Autodesk Inventor part; units mm, degrees
ref_plane "YZ Plane" through (0, 0, 0) normal (1, 0, 0) x (0, 1, 0)
ref_plane "XZ Plane" through (0, 0, 0) normal (0, 1, 0) x (-1, 0, 0)
ref_plane "XY Plane" through (0, 0, 0) normal (0, 0, 1) x (1, 0, 0)
sketch "Sketch1" plane through (0, 0, 0) normal (0, 1, 0) x (-1, 0, 0)
  line L0 (32.65, 55) -> (-32.65, 55)
  line L1 (-32.65, 55) -> (-32.65, -55)
  line L2 (-32.65, -55) -> (32.65, -55)
  line L3 (32.65, -55) -> (32.65, 55)
  line L4 (32.65, 55) -> (-32.65, -55) construction
  line L5 (-32.65, 55) -> (32.65, -55) construction
  circle A0 centre (-24.15, 38) radius 1.75
  circle A1 centre (-24.15, -45) radius 1.75
  circle A2 centre (24.15, 37) radius 1.75
  circle A3 centre (24.15, -38) radius 1.75
  point P0 (0, 0)
  dimension "d0" = 110
  dimension "d1" = 65.3
  dimension "d2" = 83
  dimension "d3" = 8.5
  dimension "d4" = 17
  dimension "d5" = 3.5
  dimension "d6" = 3.5
  dimension "d7" = 3.5
  dimension "d8" = 1
  dimension "d9" = 48.3
  dimension "d10" = 3.5
  dimension "d11" = 75
extrude "Extrusion1" add sketch "Sketch1" along normal blind 2
sketch "Sketch2" plane through (-32.65, 0, 55) normal (0, 0, 1) x (1, 0, 0)
  line L0 (0, 70) -> (65.3, 70)
  line L1 (65.3, 70) -> (65.3, 0)
  line L2 (65.3, 0) -> (0, 0)
  line L3 (0, 0) -> (0, 70)
  line L4 (0, 70) -> (65.3, 0) construction
  line L5 (65.3, 70) -> (0, 0) construction
  line L6 (65.3, 0) -> (65.3, 2)
  line L7 (16, 7.5) -> (24.5, 7.5)
  line L8 (24.5, 7.5) -> (24.5, 4)
  line L9 (24.5, 4) -> (16, 4)
  line L10 (16, 4) -> (16, 7.5)
  line L11 (16, 7.5) -> (24.5, 4) construction
  line L12 (24.5, 7.5) -> (16, 4) construction
  line L13 (32.4, 7.5) -> (40.9, 7.5)
  line L14 (40.9, 7.5) -> (40.9, 4)
  line L15 (40.9, 4) -> (32.4, 4)
  line L16 (32.4, 4) -> (32.4, 7.5)
  line L17 (32.4, 7.5) -> (40.9, 4) construction
  line L18 (40.9, 7.5) -> (32.4, 4) construction
  line L19 (45.9, 15.3) -> (55.2, 15.3)
  line L20 (55.2, 15.3) -> (55.2, 4)
  line L21 (55.2, 4) -> (45.9, 4)
  line L22 (45.9, 4) -> (45.9, 15.3)
  line L23 (45.9, 15.3) -> (55.2, 4) construction
  line L24 (55.2, 15.3) -> (45.9, 4) construction
  line L25 (0, 2) -> (65.3, 2)
  point P0 (32.65, 0)
  point P1 (32.65, 35)
  point P2 (20.25, 5.75)
  point P3 (36.65, 5.75)
  point P4 (50.55, 9.65)
  point P5 (45.9, 9.65)
  dimension "d14" = 70
  dimension "d15" = 11.3
  dimension "d16" = 9.3
  dimension "d17" = 8.5
  dimension "d18" = 3.5
  dimension "d19" = 8.5
  dimension "d20" = 3.5
  dimension "d21" = 2
  dimension "d22" = 7.9
  dimension "d23" = 16
  dimension "d24" = 5
extrude "Extrusion2" add sketch "Sketch2" against normal blind 2 contours L0 L1 L25 L3
sketch "Sketch3" plane through (32.65, 0, 55) normal (1, 0, 0) x (0, 0, -1)
  line L0 (110, 0) -> (110, 2)
  line L1 (0, 70) -> (110, 70)
  line L2 (110, 70) -> (110, 0)
  line L3 (110, 0) -> (0, 0)
  line L4 (0, 0) -> (0, 70)
  line L5 (0, 70) -> (110, 0) construction
  line L6 (110, 70) -> (0, 0) construction
  point P0 (55, 0)
  point P1 (55, 35)
  point P2 (0, 70)
extrude "Extrusion3" add sketch "Sketch3" against normal blind 2
sketch "Sketch4" plane through (-32.65, 0, -55) normal (-1, 0, 0) x (0, 0, 1)
  line L0 (110, 0) -> (110, 70)
  line L1 (0, 70) -> (110, 70)
  line L2 (110, 70) -> (110, 0)
  line L3 (110, 0) -> (0, 0)
  line L4 (0, 0) -> (0, 70)
  line L5 (0, 70) -> (110, 0) construction
  line L6 (110, 70) -> (0, 0) construction
  point P0 (55, 0)
  point P1 (55, 35)
  point P2 (0, 70)
extrude "Extrusion4" add sketch "Sketch4" against normal blind 2
sketch "Sketch5" plane through (32.65, 0, -55) normal (0, 0, -1) x (-1, 0, 0)
  line L0 (65.3, 0) -> (65.3, 70)
  line L1 (0, 70) -> (65.3, 70)
  line L2 (65.3, 70) -> (65.3, 0)
  line L3 (65.3, 0) -> (0, 0)
  line L4 (0, 0) -> (0, 70)
  line L5 (0, 70) -> (65.3, 0) construction
  line L6 (65.3, 70) -> (0, 0) construction
  line L7 (13.5, 60.35) -> (20.2, 60.35)
  line L8 (20.2, 60.35) -> (20.2, 53.65)
  line L9 (20.2, 53.65) -> (13.5, 53.65)
  line L10 (13.5, 53.65) -> (13.5, 60.35)
  line L11 (13.5, 60.35) -> (20.2, 53.65) construction
  line L12 (20.2, 60.35) -> (13.5, 53.65) construction
  line L13 (39.1, 60.35) -> (45.8, 60.35)
  line L14 (45.8, 60.35) -> (45.8, 53.65)
  line L15 (45.8, 53.65) -> (39.1, 53.65)
  line L16 (39.1, 53.65) -> (39.1, 60.35)
  line L17 (39.1, 60.35) -> (45.8, 53.65) construction
  line L18 (45.8, 60.35) -> (39.1, 53.65) construction
  line L19 (2, 2) -> (63.3, 2)
  point P0 (32.65, 0)
  point P1 (32.65, 35)
  point P2 (16.85, 57)
  point P3 (42.45, 57)
  point P4 (20.2, 57)
  point P5 (39.1, 57)
  point P6 (45.8, 57)
  dimension "d31" = 6.7
  dimension "d32" = 6.7
  dimension "d33" = 6.7
  dimension "d34" = 6.7
  dimension "d35" = 18.9
  dimension "d36" = 13.5
  dimension "d38" = 55
  dimension "d39" = 19.5
extrude "Extrusion5" add sketch "Sketch5" against normal blind 2
sketch "Sketch6" plane through (0, 0, 0) normal (0, -1, 0) x (1, 0, 0)
  line L0 (-32.65, -55) -> (32.65, -55)
  line L1 (-24.65, -63) -> (-32.65, -63)
  line L2 (-32.65, -63) -> (-32.65, -55)
  line L3 (-32.65, -55) -> (-24.65, -55)
  line L4 (-24.65, -55) -> (-24.65, -63)
  line L5 (-24.65, -63) -> (-32.65, -55) construction
  line L6 (-32.65, -63) -> (-24.65, -55) construction
  line L7 (0, 0) -> (-42.6536, 0) construction
  line L8 (0, 0) -> (0, 77.6951) construction
  line L9 (-24.65, 63) -> (-32.65, 63)
  line L10 (-32.65, 63) -> (-32.65, 55)
  line L11 (-32.65, 55) -> (-24.65, 55)
  line L12 (-24.65, 55) -> (-24.65, 63)
  line L13 (-24.65, 63) -> (-32.65, 55) construction
  line L14 (-32.65, 63) -> (-24.65, 55) construction
  line L15 (24.65, -63) -> (32.65, -63)
  line L16 (32.65, -63) -> (32.65, -55)
  line L17 (32.65, -55) -> (24.65, -55)
  line L18 (24.65, -55) -> (24.65, -63)
  line L19 (24.65, -63) -> (32.65, -55) construction
  line L20 (32.65, -63) -> (24.65, -55) construction
  line L21 (24.65, 63) -> (32.65, 63)
  line L22 (32.65, 63) -> (32.65, 55)
  line L23 (32.65, 55) -> (24.65, 55)
  line L24 (24.65, 55) -> (24.65, 63)
  line L25 (24.65, 63) -> (32.65, 55) construction
  line L26 (32.65, 63) -> (24.65, 55) construction
  circle A0 centre (-28.65, -59) radius 1.75
  circle A1 centre (-28.65, 59) radius 1.75
  circle A2 centre (28.65, -59) radius 1.75
  circle A3 centre (28.65, 59) radius 1.75
  point P0 (-28.65, 59)
  point P1 (28.65, 59)
  dimension "d42" = 8
  dimension "d43" = 8
  dimension "d44" = 3.5
extrude "Extrusion6" add sketch "Sketch6" against normal blind 2
sketch "Sketch7" plane through (0, 0, 0) normal (0, -1, 0) x (1, 0, 0)
  circle A0 centre (-24.15, -38) radius 1.75
  line L0 (-24.15, -34.6514) -> (-21.25, -36.3257)
  line L1 (-21.25, -36.3257) -> (-21.25, -39.6743)
  line L2 (-21.25, -39.6743) -> (-24.15, -41.3486)
  line L3 (-24.15, -41.3486) -> (-27.05, -39.6743)
  line L4 (-27.05, -39.6743) -> (-27.05, -36.3257)
  line L5 (-27.05, -36.3257) -> (-24.15, -34.6514)
  circle A1 centre (-24.15, 37) radius 1.75
  line L6 (-24.15, 40.3486) -> (-21.25, 38.6743)
  line L7 (-21.25, 38.6743) -> (-21.25, 35.3257)
  line L8 (-21.25, 35.3257) -> (-24.15, 33.6514)
  line L9 (-24.15, 33.6514) -> (-27.05, 35.3257)
  line L10 (-27.05, 35.3257) -> (-27.05, 38.6743)
  line L11 (-27.05, 38.6743) -> (-24.15, 40.3486)
  circle A2 centre (24.15, 38) radius 1.75
  line L12 (24.15, 41.3486) -> (27.05, 39.6743)
  line L13 (27.05, 39.6743) -> (27.05, 36.3257)
  line L14 (27.05, 36.3257) -> (24.15, 34.6514)
  line L15 (24.15, 34.6514) -> (21.25, 36.3257)
  line L16 (21.25, 36.3257) -> (21.25, 39.6743)
  line L17 (21.25, 39.6743) -> (24.15, 41.3486)
  circle A3 centre (24.15, -45) radius 1.75
  line L18 (24.15, -41.6514) -> (27.05, -43.3257)
  line L19 (27.05, -43.3257) -> (27.05, -46.6743)
  line L20 (27.05, -46.6743) -> (24.15, -48.3486)
  line L21 (24.15, -48.3486) -> (21.25, -46.6743)
  line L22 (21.25, -46.6743) -> (21.25, -43.3257)
  line L23 (21.25, -43.3257) -> (24.15, -41.6514)
  circle A4 centre (-28.65, 59) radius 1.75
  circle A5 centre (28.65, -59) radius 1.75
  circle A6 centre (28.65, 59) radius 1.75
  circle A7 centre (-28.65, -59) radius 1.75
  circle A8 centre (-24.15, -38) radius 1.75
  circle A9 centre (-24.15, 37) radius 1.75
  circle A10 centre (24.15, -45) radius 1.75
  circle A11 centre (24.15, 38) radius 1.75
  line L24 (32.65, 63) -> (32.65, -63)
  line L25 (32.65, 63) -> (24.65, 63)
  line L26 (24.65, 63) -> (24.65, 55)
  line L27 (-24.65, 55) -> (24.65, 55)
  line L28 (-24.65, 55) -> (-24.65, 63)
  line L29 (-24.65, 63) -> (-32.65, 63)
  line L30 (-32.65, 63) -> (-32.65, -63)
  line L31 (-32.65, -63) -> (-24.65, -63)
  line L32 (-24.65, -63) -> (-24.65, -55)
  line L33 (24.65, -55) -> (-24.65, -55)
  line L34 (24.65, -55) -> (24.65, -63)
  line L35 (24.65, -63) -> (32.65, -63)
  point P0 (0, 0)
  point P1 (27.05, 38)
  point P2 (21.25, 38)
  point P3 (27.05, -45)
  point P4 (21.25, -45)
  dimension "d47" = 5.8
  dimension "d48" = 5.8
  dimension "d49" = 5.8
  dimension "d50" = 5.8
extrude "Extrusion7" add sketch "Sketch7" along normal blind 2.5 contours L24 L35 L34 L33 L32 L31 L30 L29 L28 L27 L26 L25
equation "\"d6\" = d5"
equation "\"d7\" = d5"
equation "\"d10\" = d5"
equation "\"d48\" = d47"
properties part number "base"
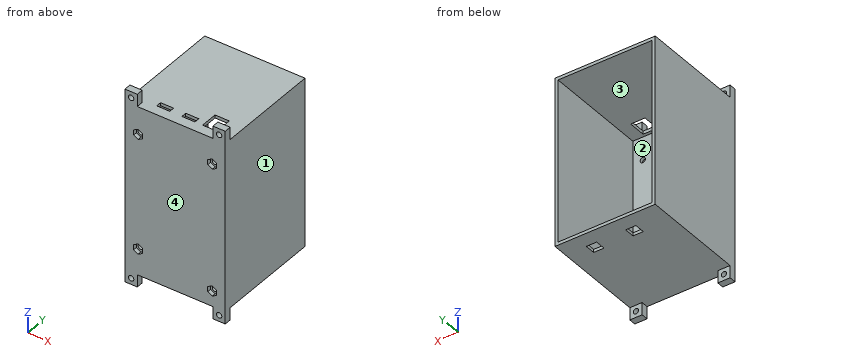
For this review, take the finished solid that the model builds, in its own axes (mm). Face numbers are marked on the shaded views. A direction names the side the tool comes from. Coordinates: 2 decimals unless noted, no trailing zeros. Loops run counter-clockwise (first coordinate to the right, second up) from the corner with the lowest first, then second, coordinate; pieces in that order, holes last. Notation, with made-up numbers: (73, 57) - (80, 57) arc R12 ccw to (80, 79) - close; hole circle Ø7 at (89.5, 82.5). An arc over 180 degrees is marked (long way). Use a Markdown table: item, result. Add a question column.
Item 1: Tool access review of the marked faces 3 and 4: name each direction out of +Z, -Z, +X, -X, +Y, -Y from which nothing blocks a thin tool from reaching the whole face with its end or side.
Item 2: For line 1 (Z direction, x = -28.65, y = 1.1); line 2 (Z direction, x = 24.15, y = 0.4); line 3 (Z direction, x = 14.5, y = 19.5), list the stretches that pass through material, from the lowest coordinate up.
Item 3: We need section D-D (z = -45). Give the boundary of the cut face in (x, y).
Item 4: We need section C-C (y = 52). Give the boundary of the cut face in (x, z), and give its area (3 significant figures).
Item 5: We need section B-B (x = 28.65). Give the boundary of the cut face in (y, z).
Item 6: Mouldability with a two-part tool opening along Z and no side actions: class the marked faces 1 and 2 as pulls with the +Z half, pulls with the -Z half, needs draft (parallel to the pull), parting line crosses it, or undercut.
Item 7: We need section A-A (z = -59). Give the boundary of the cut face in (x, y).
Item 8: Insertion check: pin 1 Ø4 at (x, z) = (-28.65, -59) entering from +Y; pin 2 Ø8 at (x, y) = (-13.5, 32) entering from -Z; pin 3 Ø3 at (x, z) = (28.65, -59) entering from -Y; pin 4 Ø6.5 at (x, z) = (-24.5, 37.5) entering from -Y. Each pin has a flat end and moves straight along its axis. Give the tip position at first contact, or say it passes through.
Results list:
| question | item | result |
|---|---|---|
| 1 | face 3 | +Y |
| 1 | face 4 | +Z, -Z, +X, -X, -Y |
| 2 | line 1 | z = -63 to -60.75, -57.25 to 57.25, 60.75 to 63 |
| 2 | line 2 | z = -55 to -46.75, -43.25 to 36.25, 39.75 to 55 |
| 2 | line 3 | z = -55 to -53, 53 to 55 |
| 3 | outline | (-32.65, -2.5) - (21.25, -2.5) - (21.25, 0) - (22.4, 0) - (22.4, 2) - (-30.65, 2) - (-30.65, 70) - (-32.65, 70) - close; (25.9, 0) - (27.05, 0) - (27.05, -2.5) - (32.65, -2.5) - (32.65, 70) - (30.65, 70) - (30.65, 2) - (25.9, 2) - close |
| 4 | outline | (-32.65, -55) - (32.65, -55) - (32.65, 55) - (-32.65, 55) - close; hole (-30.65, -53) - (30.65, -53) - (30.65, 53) - (-30.65, 53) - close |
| 4 | area | 685 mm^2 |
| 5 | outline | (-2.5, -63) - (2, -63) - (2, -60.75) - (-2.5, -60.75) - close; (-2.5, -57.25) - (2, -57.25) - (2, -55) - (70, -55) - (70, -53) - (2, -53) - (2, 53) - (70, 53) - (70, 55) - (2, 55) - (2, 57.25) - (-2.5, 57.25) - close; (-2.5, 60.75) - (2, 60.75) - (2, 63) - (-2.5, 63) - close |
| 6 | face 1 | needs draft |
| 6 | face 2 | undercut |
| 7 | outline | (-32.65, -2.5) - (-30.4, -2.5) - (-30.4, 2) - (-32.65, 2) - close; (-26.9, -2.5) - (-24.65, -2.5) - (-24.65, 2) - (-26.9, 2) - close; (24.65, -2.5) - (26.9, -2.5) - (26.9, 2) - (24.65, 2) - close; (30.4, -2.5) - (32.65, -2.5) - (32.65, 2) - (30.4, 2) - close |
| 8 | pin 1 | stops at y = 2 |
| 8 | pin 2 | stops at z = -55 |
| 8 | pin 3 | passes through |
| 8 | pin 4 | stops at y = -2.5 |
